Job drawing, mm, ordinate dimensions from the low corner. One solid piece. A direction names the side the tool comes from. Round coordinates to 2 decimals unless told otherwise and drop trailing zeros. Write each loop counter-clockwise with the first axis right and the second up, starting at its lowest first coordinate (ties: lowest second). Pieces come first, ordered by that corner, then holes.
1) Flat gauge pins, fed straight in: pin 1 (2.5 mm diameter, centred on y = 17, z = 5, fed in from +X); pin 2 (4 mm diameter, centred on y = 15, z = 23, fed in from -X); pin 3 (1.5 mm diameter, centred on x = 38, z = 27.5, fed in from +Y); pin 4 (10 mm diameter, centred on x = 21, z = 26.5, fed in from -Y). Where does each tip first touch, or does it go through?
2) Pull direction X, two halves, no side cores. Call the marked faces 1, 2 and 3: +X half, -X half, draft (parallel to the pull), parting line (faces both ways), or undercut.
3) Saw through at C-C (x = 49.5). Write the cut outline in (y, z).
4) Saw through at B-B (z = 20.5). Write the cut outline in (x, y).
5) Which spindle directions (+Z, -Z, +X, -X, +Y, -Y) get a long thin tool onto all of the face, cutting with end or side? Do the marked faces 4, 5, 6, 7 and 8. Say none if no direction does.
6) Saw through at A-A (y = 18). Write the cut outline in (x, z), plus the area to 3 significant figures.
7) Wall check: probe 1 along Z at (x, y) = (53, 17.5); probe 2 along Y at (x, z) = (54, 11); probe 3 along X at (y, z) = (11, 29). Give the ranges that are in metal, low to high.
8) Saw through at D-D (y = 25.5). Write the cut outline in (x, z).
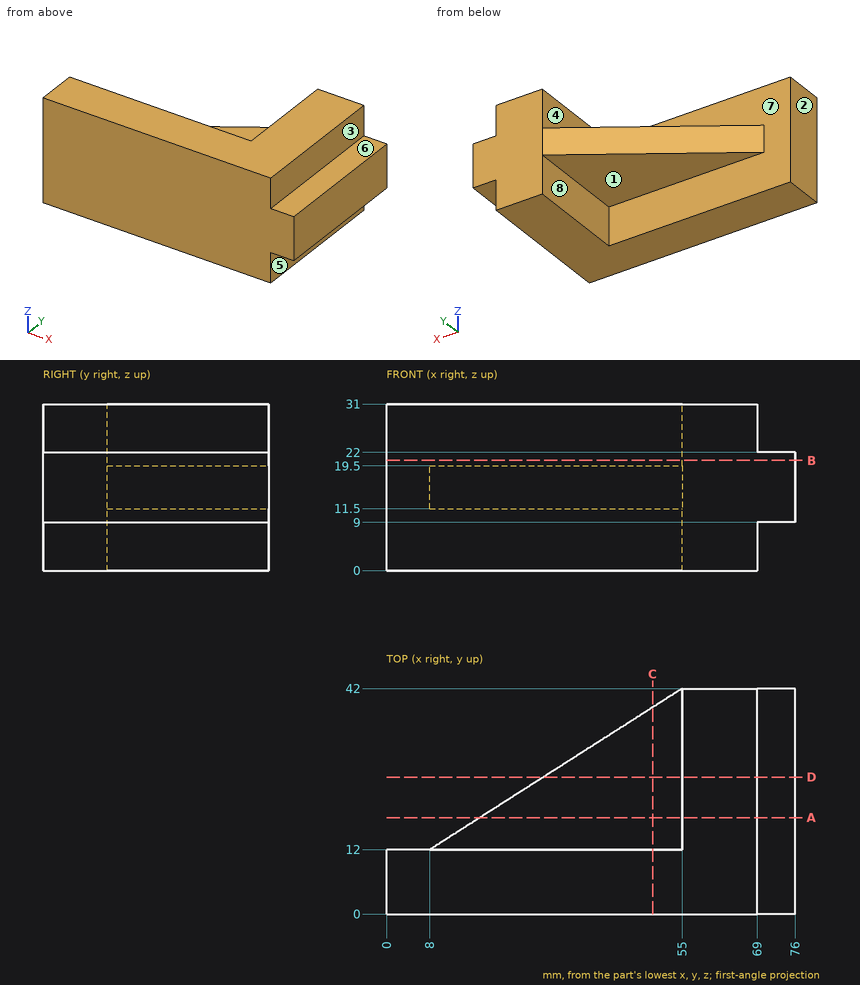
Evaluation:
1. pin 1: stops at x = 69
1. pin 2: stops at x = 55
1. pin 3: stops at y = 12
1. pin 4: stops at y = 0
2. face 1: draft
2. face 2: -X half
2. face 3: +X half
3. outline: (0, 0) - (12, 0) - (12, 11.5) - (38.49, 11.5) - (38.49, 19.5) - (12, 19.5) - (12, 31) - (0, 31) - close
4. outline: (0, 0) - (76, 0) - (76, 42) - (55, 42) - (55, 12) - (0, 12) - close
5. face 4: +Z, -X, +Y
5. face 5: -Z, +X, +Y, -Y
5. face 6: +Z, +X, +Y, -Y
5. face 7: -X, +Y
5. face 8: -Z, -X, +Y
6. outline: (17.4, 11.5) - (55, 11.5) - (55, 0) - (69, 0) - (69, 9) - (76, 9) - (76, 22) - (69, 22) - (69, 31) - (55, 31) - (55, 19.5) - (17.4, 19.5) - close
6. area: 826 mm2
7. probe 1: z = 11.5 to 19.5
7. probe 2: y = 0 to 12
7. probe 3: x = 0 to 69
8. outline: (29.15, 11.5) - (55, 11.5) - (55, 0) - (69, 0) - (69, 9) - (76, 9) - (76, 22) - (69, 22) - (69, 31) - (55, 31) - (55, 19.5) - (29.15, 19.5) - close
